Autodesk Inventor part; units mm, degrees
ref_plane "YZ Plane" through (0, 0, 0) normal (1, 0, 0) x (0, 1, 0)
ref_plane "XZ Plane" through (0, 0, 0) normal (0, 1, 0) x (-1, 0, 0)
ref_plane "XY Plane" through (0, 0, 0) normal (0, 0, 1) x (1, 0, 0)
sketch "Boceto1" plane through (0, 0, 0) normal (0, 1, 0) x (-1, 0, 0)
  arc A0 (56.9996, -30) -> (66.9996, -30) centre (61.9996, -30) ccw
  circle A1 centre (62, 0) radius 1.5
  circle A2 centre (61.9996, 8) radius 1.5
  circle A3 centre (62, -8) radius 1.5
  line L0 (69.9996, 8) -> (66.9996, -30)
  line L1 (53.9996, 8) -> (56.9996, -30)
  arc A4 (69.9996, 8) -> (53.9996, 8) centre (61.9996, 8) ccw
  circle A5 centre (61.9996, -30) radius 1.5
  dimension "d126" = 3
extrude "Extrusión1" add sketch "Boceto1" along normal blind 3
properties part number "manivela"
Check sheet for the modelled part. Datum: model origin and axes. Units: mm. Give positions to 0.01 mm unless a question says otherwise; leave off trailing zeros. Write each loop counter-clockwise with the first axis right and the second up, starting at its lowest first coordinate (ties: lowest second). Pieces come first, ordered by that corner, then holes.
Item 1: Cross-section at B-B (z = 0). Enter the section's corners in (x, y).
Item 2: Draft check along Z on faces 1 (the face through (-64, 0, -9)), 2 (the face through (-62, 1, -35)), 3 (the face through (-62, 1, 16)), 4 (the face through (-63.386, 1.479, -7.425)). Enter one of: released by +Z, released by -Z, zero draft, split by the parting line, or undercut.
Item 3: Cross-section at D-D (z = -7). Enter the section's corners in (x, y), and give its area (3 significant figures).
Item 4: Cross-section at C-C (y = 1.45). Enter the section's corners in (x, z), and give its area (3 significant figures).
Item 5: Gauge pin test, flat ends, axial feed: pin 1 (4 mm diameter, centred on x = -65, z = 5.5, fed in from -Y); pin 2 (1.5 mm diameter, centred on y = 2, z = -18, fed in from +X). Record the tip position at first contact, or that the pin passes through.
Item 6: Cross-section at A-A (x = -62). Enter the section's corners in (y, z).
Item 7: Scan lines: L1, parallel to Z at x = -62, y = 0.8; L2, parallel to X at y = 2.3, z = 1; L3, parallel to Z at x = -60.25, y = 0.5. Record each from-to range of solid material in increasing order.
Report:
1. outline: (-69.37, 0) - (-63.5, 0) - (-63.5, 3) - (-69.37, 3) - close; (-60.5, 0) - (-54.63, 0) - (-54.63, 3) - (-60.5, 3) - close
2. face 1: zero draft
2. face 2: released by -Z
2. face 3: released by +Z
2. face 4: undercut
3. outline: (-68.82, 0) - (-63.12, 0) - (-63.12, 3) - (-68.82, 3) - close; (-60.88, 0) - (-55.18, 0) - (-55.18, 3) - (-60.88, 3) - close
3. area: 34.2 mm2
4. outline: (-70, 8) - (-67, -30) arc R5 ccw to (-57, -30) - (-54, 8) arc R8 ccw to start; hole circle Ø3 at (-62, -30); hole circle Ø3 at (-62, -8); hole circle Ø3 at (-62, 0); hole circle Ø3 at (-62, 8)
4. area: 606 mm2
5. pin 1: stops at y = 0
5. pin 2: stops at x = -55.99
6. outline: (0, -35) - (3, -35) - (3, -31.5) - (0, -31.5) - close; (0, -28.5) - (3, -28.5) - (3, -9.5) - (0, -9.5) - close; (0, -6.5) - (3, -6.5) - (3, -1.5) - (0, -1.5) - close; (0, 1.5) - (3, 1.5) - (3, 6.5) - (0, 6.5) - close; (0, 9.5) - (3, 9.5) - (3, 16) - (0, 16) - close
7. L1: z = -35 to -31.5, -28.5 to -9.5, -6.5 to -1.5, 1.5 to 6.5, 9.5 to 16
7. L2: x = -69.45 to -63.12, -60.88 to -54.55
7. L3: z = -34.68 to 15.81
